from build123d import *

# Parameters (mm, degrees)
F0_W     = 622.3
F0_H     = 531.8125
F0_R     = 2.413
F0_R_2   = 4.7625
F0_W_2   = 210.82
F0_H_2   = 310.388
F1_DEPTH = 25.4
F2_T     = -2.54
F3_W     = 617.22
F3_H     = 22.86
F4_DEPTH = 526.7325


with BuildPart() as f1:
    # F0 (on Front) → F1 (new body)
    with BuildSketch(Plane.XZ):
        with Locations((0, 265.90625)):
            Rectangle(F0_W, F0_H)
        with Locations((-190.5, 54.483)):
            Circle(F0_R, mode=Mode.SUBTRACT)
        with Locations((-292.1, 95.25)):
            Circle(F0_R_2, mode=Mode.SUBTRACT)
        with Locations((-259.588, 91.694)):
            Circle(F0_R, mode=Mode.SUBTRACT)
        with Locations((-88.9, 54.483)):
            Circle(F0_R, mode=Mode.SUBTRACT)
        with Locations((-19.812, 91.694)):
            Circle(F0_R, mode=Mode.SUBTRACT)
        with Locations((-259.588, 174.244)):
            Circle(F0_R, mode=Mode.SUBTRACT)
        with Locations((-19.812, 174.244)):
            Circle(F0_R, mode=Mode.SUBTRACT)
        with Locations((-139.7, 225.044)):
            Rectangle(F0_W_2, F0_H_2, mode=Mode.SUBTRACT)
        with Locations((88.9, 54.483)):
            Circle(F0_R, mode=Mode.SUBTRACT)
        with Locations((19.812, 91.694)):
            Circle(F0_R, mode=Mode.SUBTRACT)
        with Locations((190.5, 54.483)):
            Circle(F0_R, mode=Mode.SUBTRACT)
        with Locations((259.588, 91.694)):
            Circle(F0_R, mode=Mode.SUBTRACT)
        with Locations((292.1, 95.25)):
            Circle(F0_R_2, mode=Mode.SUBTRACT)
        with Locations((19.812, 174.244)):
            Circle(F0_R, mode=Mode.SUBTRACT)
        with Locations((139.7, 225.044)):
            Rectangle(F0_W_2, F0_H_2, mode=Mode.SUBTRACT)
        with Locations((259.588, 174.244)):
            Circle(F0_R, mode=Mode.SUBTRACT)
        with Locations((-259.588, 275.844)):
            Circle(F0_R, mode=Mode.SUBTRACT)
        with Locations((-259.588, 358.394)):
            Circle(F0_R, mode=Mode.SUBTRACT)
        with Locations((-190.5, 395.605)):
            Circle(F0_R, mode=Mode.SUBTRACT)
        with Locations((-19.812, 275.844)):
            Circle(F0_R, mode=Mode.SUBTRACT)
        with Locations((-88.9, 395.605)):
            Circle(F0_R, mode=Mode.SUBTRACT)
        with Locations((-19.812, 358.394)):
            Circle(F0_R, mode=Mode.SUBTRACT)
        with Locations((-292.1, 438.15)):
            Circle(F0_R_2, mode=Mode.SUBTRACT)
        with Locations((19.812, 275.844)):
            Circle(F0_R, mode=Mode.SUBTRACT)
        with Locations((19.812, 358.394)):
            Circle(F0_R, mode=Mode.SUBTRACT)
        with Locations((88.9, 395.605)):
            Circle(F0_R, mode=Mode.SUBTRACT)
        with Locations((259.588, 275.844)):
            Circle(F0_R, mode=Mode.SUBTRACT)
        with Locations((190.5, 395.605)):
            Circle(F0_R, mode=Mode.SUBTRACT)
        with Locations((259.588, 358.394)):
            Circle(F0_R, mode=Mode.SUBTRACT)
        with Locations((292.1, 438.15)):
            Circle(F0_R_2, mode=Mode.SUBTRACT)
    extrude(amount=F1_DEPTH)

    # F2
    f2_openings = [f1.faces().sort_by_distance(p)[0] for p in [
        (0, 0, 292.820788),
    ]]
    offset(amount=F2_T, openings=f2_openings, kind=Kind.INTERSECTION)

    # F3 (on face) → F4 (cut, through all)
    with BuildSketch(Plane(origin=(0, 0, 529.2725), x_dir=(1, 0, 0), z_dir=(0, 0, -1))):
        with Locations((0, 11.43)):
            Rectangle(F3_W, F3_H)
    extrude(amount=F4_DEPTH, mode=Mode.SUBTRACT)


solid = f1.part
Verification items for the finished model (mm, model axes). A direction names the side the tool comes from. Give positions to 0.01 mm unless a question says otherwise; leave off trailing zeros. Loops run counter-clockwise (first coordinate to the right, second up) from the corner with the lowest first, then second, coordinate; pieces in that order, holes last. Notation, with made-up numbers: (-30.5, -32) - (-1.5, -32) arc R5 cw to (-1.5, -27) - close; hole circle Ø9 at (68.5, 55.25). An arc over 180 degrees is marked (long way). Write each question's results on one line, items separated by ' | '.
1) Sectioned sample at C-C on z = 189. Record the boundary of the cut face in (x, y).
Solution:
outline: (-311.15, -25.4) - (-245.11, -25.4) - (-245.11, -22.86) - (-308.61, -22.86) - (-308.61, 0) - (-311.15, 0) - close; (-34.29, -25.4) - (34.29, -25.4) - (34.29, -22.86) - (-34.29, -22.86) - close; (245.11, -25.4) - (311.15, -25.4) - (311.15, 0) - (308.61, 0) - (308.61, -22.86) - (245.11, -22.86) - close
2) Sectioned sample at D-D on z = 493.5. Record the boundary of the cut face in (x, y), plus the area to 3 significant figures.
Solution:
outline: (-311.15, -25.4) - (311.15, -25.4) - (311.15, 0) - (308.61, 0) - (308.61, -22.86) - (-308.61, -22.86) - (-308.61, 0) - (-311.15, 0) - close | area: 1,700 mm2
3) Sectioned sample at A-A on x = -216. Record the boundary of the cut face in (y, z), plus the area to 3 significant figures.
Solution:
outline: (-25.4, 0) - (0, 0) - (0, 2.54) - (-22.86, 2.54) - (-22.86, 69.85) - (-25.4, 69.85) - close; (-25.4, 380.24) - (-22.86, 380.24) - (-22.86, 529.27) - (0, 529.27) - (0, 531.81) - (-25.4, 531.81) - close | area: 679 mm2
4) Tool access check on faces 4 (the flat face through (-4, -25.4, 329)), 5 (the flat face through (-4, -22.86, 328)). Record the directions out of +Z, -Z, +X, -X, +Y, -Y that give a thin tool (end or side, any length) a straight path to the whole face; none if there is none.
Solution:
face 4: +Z, -Z, +X, -X, -Y | face 5: +Y
5) Mould release check, pull along Z, two halves, no side actions. Record for faces 1 (the flat face through (-4, -13, 0)), 2 (the flat face through (-4, -13, 531.812)), 3 (the flat face through (308.61, -11, 262)): pulls with the +Z half, pulls with the -Z half, needs draft (parallel to the pull), parting line crosses it, or undercut.
Solution:
face 1: pulls with the -Z half | face 2: pulls with the +Z half | face 3: undercut
6) Sectioned sample at B-B on y = -7.5. Record the boundary of the cut face in (x, z), plus the area to 3 significant figures.
Solution:
outline: (-311.15, 0) - (311.15, 0) - (311.15, 531.81) - (-311.15, 531.81) - close; hole (-308.61, 2.54) - (308.61, 2.54) - (308.61, 529.27) - (-308.61, 529.27) - close | area: 5,840 mm2
7) Material ranges on L1, parallel to X at y = -24.35, z = 95.25; L2, parallel to Z at x = -292.1, y = -24.8; L3, parallel to X at y = -20, z = 51, recorded low to high. Write a range as from..to.
Solution:
L1: -311.15..-296.86, -287.34..-245.11, -34.29..34.29, 245.11..287.34, 296.86..311.15 | L2: 0..90.49, 100.01..433.39, 442.91..531.81 | L3: -311.15..-308.61, 308.61..311.15
8) Depth check by flat-ended pin: P1, Ø12.5, axis at x = -292.1, z = 438.15, coming from the +Y side; P2, Ø4, axis at x = 88.9, z = 54.483, coming from the +Y side; P3, Ø6, axis at x = 57.5, y = -22, coming from the -Z side. Enter the tip coordinate at first touch or a pass-through.
Solution:
P1: y = -22.86 | P2: through | P3: z = 0
